Could you check a few things on this model? Use its own coordinates, in mm. Give positions to 0.01 mm unless a question says otherwise; leave off trailing zeros.
1. Imagine slicing it at A-A (y = 0.5). Count the separate pieces of the cut face and the enclosed holes in it, plus the area to 3 significant figures.
2. For P1, Ø2, axis at x = 420, z = 78, coming from the -Y side, with a flat end and sliding along its axis, tell me the tip position at first contact or that it passes through.
3. I need wall thicknesses on line 1 along Z through (x, y) = (553.5, 1.35); line 2 along Z through (x, y) = (452, 0.1); line 3 along X through (y, z) = (0.1, 67.5). Which ranges of each line are inside material? Lowest first, please.
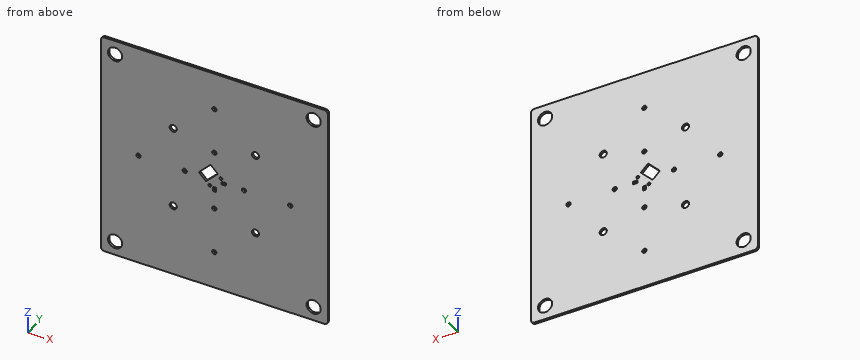
```python
from build123d import *

# Parameters (mm, degrees)
SKETCH1_R           = 5
SKETCH1_R_2         = 1.525
SKETCH1_R_3         = 2.525
SKETCH1_R_4         = 1.025
BOSS_EXTRUDE1_DEPTH = 1.6


with BuildPart() as part:
    # Sketch1 → Boss-Extrude1 (new body)
    with BuildSketch(Plane(origin=(0, 0, 0), x_dir=(1, 0, 0), z_dir=(0, 1, 0))):
        with BuildLine():
            Line((557.234258902, 42.261494271), (402.234258902, 42.261494271))
            ThreePointArc((402.234258902, 42.261494271), (400.466491949, 41.529261224), (399.734258902, 39.761494271))
            Line((399.734258902, 39.761494271), (399.734258902, -115.238505729))
            ThreePointArc((399.734258902, -115.238505729), (400.466491949, -117.006272682), (402.234258902, -117.738505729))
            Line((402.234258902, -117.738505729), (557.234258902, -117.738505729))
            ThreePointArc((557.234258902, -117.738505729), (559.002025855, -117.006272682), (559.734258902, -115.238505729))
            Line((559.734258902, -115.238505729), (559.734258902, 39.761494271))
            ThreePointArc((559.734258902, 39.761494271), (559.002025855, 41.529261224), (557.234258902, 42.261494271))
        make_face()
        with Locations(Location((409.734258902, -107.738505729, 0), (0, 0, 270))):
            Circle(SKETCH1_R, mode=Mode.SUBTRACT)
        with Locations(Location((479.734258902, -91.238505729, 0), (0, 0, 270))):
            Circle(SKETCH1_R_2, mode=Mode.SUBTRACT)
        with Locations(Location((450.742880873, -66.729883758, 0), (0, 0, 270))):
            Circle(SKETCH1_R_3, mode=Mode.SUBTRACT)
        with Locations(Location((479.734258902, -58.638505729, 0), (0, 0, 270))):
            Circle(SKETCH1_R_2, mode=Mode.SUBTRACT)
        with BuildLine():
            Line((474.218826009, -35.617185386), (481.855579245, -43.253938622))
            ThreePointArc((481.855579245, -43.253938622), (482.002025855, -43.607492013), (481.855579245, -43.961045404))
            Line((481.855579245, -43.961045404), (477.471517202, -48.345107447))
            ThreePointArc((477.471517202, -48.345107447), (477.117963811, -48.491554056), (476.764410421, -48.345107447))
            Line((476.764410421, -48.345107447), (469.127657184, -40.70835421))
            ThreePointArc((469.127657184, -40.70835421), (468.981210575, -40.35480082), (469.127657184, -40.001247429))
            Line((469.127657184, -40.001247429), (473.511719227, -35.617185386))
            ThreePointArc((473.511719227, -35.617185386), (473.865272618, -35.470738776), (474.218826009, -35.617185386))
        make_face(mode=Mode.SUBTRACT)
        with Locations(Location((549.734258902, -107.738505729, 0), (0, 0, 270))):
            Circle(SKETCH1_R, mode=Mode.SUBTRACT)
        with Locations(Location((508.725636931, -66.729883758, 0), (0, 0, 270))):
            Circle(SKETCH1_R_3, mode=Mode.SUBTRACT)
        with Locations(Location((484.33045298, -40.920486245, 0), (0, 0, 270))):
            Circle(SKETCH1_R_4, mode=Mode.SUBTRACT)
        with Locations(Location((426.234258902, -37.738505729, 0), (0, 0, 270))):
            Circle(SKETCH1_R_2, mode=Mode.SUBTRACT)
        with Locations(Location((458.834258902, -37.738505729, 0), (0, 0, 270))):
            Circle(SKETCH1_R_2, mode=Mode.SUBTRACT)
        with Locations(Location((476.552278387, -33.142311651, 0), (0, 0, 270))):
            Circle(SKETCH1_R_4, mode=Mode.SUBTRACT)
        Polygon((480.734258902, -32.838505729), (479.734258902, -32.838505729), (478.734258902, -32.838505729), (478.734258902, -29.638505729), (480.734258902, -29.638505729), align=None, mode=Mode.SUBTRACT)
        with Locations(Location((450.742880873, -8.747127701, 0), (0, 0, 270))):
            Circle(SKETCH1_R_3, mode=Mode.SUBTRACT)
        with Locations(Location((479.734258902, -16.838505729, 0), (0, 0, 270))):
            Circle(SKETCH1_R_2, mode=Mode.SUBTRACT)
        with Locations(Location((409.734258902, 32.261494271, 0), (0, 0, 270))):
            Circle(SKETCH1_R, mode=Mode.SUBTRACT)
        with Locations(Location((479.734258902, 15.761494271, 0), (0, 0, 270))):
            Circle(SKETCH1_R_2, mode=Mode.SUBTRACT)
        Polygon((484.634258902, -38.738505729), (484.634258902, -37.738505729), (484.634258902, -36.738505729), (487.834258902, -36.738505729), (487.834258902, -38.738505729), align=None, mode=Mode.SUBTRACT)
        with Locations(Location((500.634258902, -37.738505729, 0), (0, 0, 270))):
            Circle(SKETCH1_R_2, mode=Mode.SUBTRACT)
        with Locations(Location((508.725636931, -8.747127701, 0), (0, 0, 270))):
            Circle(SKETCH1_R_3, mode=Mode.SUBTRACT)
        with Locations(Location((533.234258902, -37.738505729, 0), (0, 0, 270))):
            Circle(SKETCH1_R_2, mode=Mode.SUBTRACT)
        with Locations(Location((549.734258902, 32.261494271, 0), (0, 0, 270))):
            Circle(SKETCH1_R, mode=Mode.SUBTRACT)
    extrude(amount=BOSS_EXTRUDE1_DEPTH)


solid = part.part
```
Derived:
1. separate pieces: 1
1. enclosed holes: 21
1. area: 25,000 mm2
2. P1: stops at y = 0
3. line 1: z = -42.26 to -35.55, -28.97 to 104.45, 111.03 to 117.74
3. line 2: z = -42.26 to 6.56, 10.94 to 64.54, 68.92 to 117.74
3. line 3: x = 399.73 to 448.34, 453.15 to 506.32, 511.13 to 559.73
